Part model, mm, in its own coordinate system. Face numbers are marked on the shaded views. Round coordinates to 2 decimals unless told otherwise and drop trailing zeros. Loops run counter-clockwise (first coordinate to the right, second up) from the corner with the lowest first, then second, coordinate; pieces in that order, holes last.
1) Band-saw the part on D-D, the plane x = 15. Write the cut outline in (y, z).
2) Mould opens along Z. For the marked faces 1 and 2 say: +Z half, -Z half, draft (parallel to the pull), parting line (faces both ways), or undercut.
3) Probe line 1 (X direction, y = 4, z = -22); line 2 (X direction, y = 1.5, z = 10); line 3 (X direction, y = 5, z = -17). List the from-to ranges inside material, lowest first.
4) Band-saw the part on A-A, the plane x = 0. Write the cut outline in (y, z).
5) Drop flat-ended pins along their axis: P1, Ø2, axis at x = 0, y = 4.5, coming from the +Z side; P2, Ø4, axis at x = -20, y = 6, coming from the -Z side; P3, Ø3, axis at x = -7.5, y = 4, coming from the +Z side. Give the stop position or say it passes through.
6) Band-saw the part on C-C, the plane z = 17. Write the cut outline in (x, y), then the cut area to 3 significant figures.
7) Band-saw the part on B-B, the plane z = 0. Write the cut outline in (x, y), then the cut area to 3 significant figures.
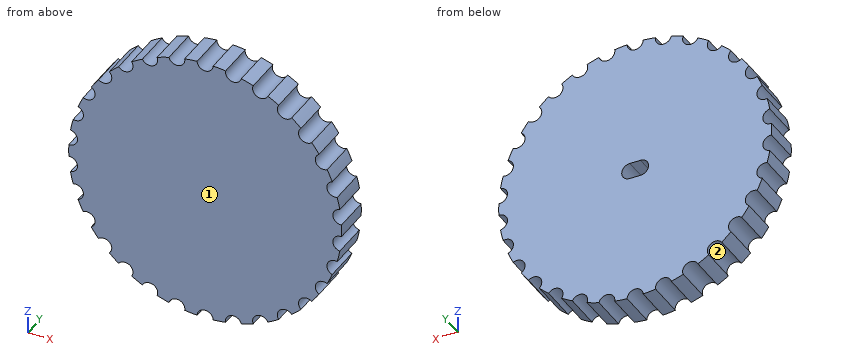
from build123d import *

# Parameters (mm, degrees)
SKETCH1_R           = 25.4
BOSS_EXTRUDE1_DEPTH = 7
CUT_EXTRUDE1_DEPTH  = 6
SKETCH4_R           = 1.496602071
CUT_EXTRUDE2_DEPTH  = 37.596721165


with BuildPart() as part:
    # Sketch1 → Boss-Extrude1 (new body)
    with BuildSketch(Plane(origin=(0, 0, 0), x_dir=(1, 0, 0), z_dir=(0, 1, 0))):
        with Locations(Location((0, 0, 0), (0, 0, 270))):
            Circle(SKETCH1_R)
    extrude(amount=BOSS_EXTRUDE1_DEPTH)

    # Sketch3 → Cut-Extrude1 (cut)
    with BuildSketch(Plane(origin=(0, 7, 0), x_dir=(1, 0, 0), z_dir=(0, 1, 0))):
        with BuildLine():
            Line((-1, 1.5), (1, 1.5))
            ThreePointArc((1, 1.5), (2.5, 0), (1, -1.5))
            Line((1, -1.5), (-1, -1.5))
            ThreePointArc((-1, -1.5), (-2.5, 0), (-1, 1.5))
        make_face()
    extrude(amount=-CUT_EXTRUDE1_DEPTH, mode=Mode.SUBTRACT)

    # Sketch4 → Cut-Extrude2 (cut, through all)
    with BuildSketch(Plane(origin=(0, 7, 0), x_dir=(1, 0, 0), z_dir=(0, 1, 0))):
        with Locations((0, 25.4)):
            Circle(SKETCH4_R)
        with Locations((5.280956947, 24.844949059)):
            Circle(SKETCH4_R)
        with Locations((10.331110734, 23.204054624)):
            Circle(SKETCH4_R)
        with Locations((14.929745408, 20.549031657)):
            Circle(SKETCH4_R)
        with Locations((18.875878567, 16.995917402)):
            Circle(SKETCH4_R)
        with Locations((21.997045256, 12.7)):
            Circle(SKETCH4_R)
        with Locations((24.156835514, 7.849031657)):
            Circle(SKETCH4_R)
        with Locations((25.260856142, 2.655022967)):
            Circle(SKETCH4_R)
        with Locations((25.260856142, -2.655022967)):
            Circle(SKETCH4_R)
        with Locations((24.156835514, -7.849031657)):
            Circle(SKETCH4_R)
        with Locations((21.997045256, -12.7)):
            Circle(SKETCH4_R)
        with Locations((18.875878567, -16.995917402)):
            Circle(SKETCH4_R)
        with Locations((14.929745408, -20.549031657)):
            Circle(SKETCH4_R)
        with Locations((10.331110734, -23.204054624)):
            Circle(SKETCH4_R)
        with Locations((5.280956947, -24.844949059)):
            Circle(SKETCH4_R)
        with Locations((0, -25.4)):
            Circle(SKETCH4_R)
        with Locations((-5.280956947, -24.844949059)):
            Circle(SKETCH4_R)
        with Locations((-10.331110734, -23.204054624)):
            Circle(SKETCH4_R)
        with Locations((-14.929745408, -20.549031657)):
            Circle(SKETCH4_R)
        with Locations((-18.875878567, -16.995917402)):
            Circle(SKETCH4_R)
        with Locations((-21.997045256, -12.7)):
            Circle(SKETCH4_R)
        with Locations((-24.156835514, -7.849031657)):
            Circle(SKETCH4_R)
        with Locations((-25.260856142, -2.655022967)):
            Circle(SKETCH4_R)
        with Locations((-25.260856142, 2.655022967)):
            Circle(SKETCH4_R)
        with Locations((-24.156835514, 7.849031657)):
            Circle(SKETCH4_R)
        with Locations((-21.997045256, 12.7)):
            Circle(SKETCH4_R)
        with Locations((-18.875878567, 16.995917402)):
            Circle(SKETCH4_R)
        with Locations((-14.929745408, 20.549031657)):
            Circle(SKETCH4_R)
        with Locations((-10.331110734, 23.204054624)):
            Circle(SKETCH4_R)
        with Locations((-5.280956947, 24.844949059)):
            Circle(SKETCH4_R)
    extrude(amount=-CUT_EXTRUDE2_DEPTH, mode=Mode.SUBTRACT)


solid = part.part
Reported:
1. outline: (0, -19.05) - (7, -19.05) - (7, 19.05) - (0, 19.05) - close
2. face 1: draft
2. face 2: undercut
3. line 1: x = -12.69 to -11.22, -9.44 to 9.44, 11.22 to 12.69
3. line 2: x = -23.35 to 23.35
3. line 3: x = -17.38 to 17.38
4. outline: (0, -23.9) - (7, -23.9) - (7, -1.5) - (1, -1.5) - (1, 1.5) - (7, 1.5) - (7, 23.9) - (0, 23.9) - close
5. P1: stops at z = 24.29
5. P2: stops at z = -15.85
5. P3: stops at z = 24.49
6. outline: (-17.38, 0) - (17.38, 0) - (17.38, 7) - (-17.38, 7) - close
6. area: 243 mm2
7. outline: (-25.4, 0) - (25.4, 0) - (25.4, 7) - (2.5, 7) - (2.5, 1) - (-2.5, 1) - (-2.5, 7) - (-25.4, 7) - close
7. area: 326 mm2
